Check sheet for the drawn part. Datum: minimum x, y, z corner. Units: mm. A direction names the side the tool comes from. Coordinates: 2 decimals unless noted, no trailing zeros. Write each loop counter-clockwise with the first axis right and the second up, starting at its lowest first coordinate (ties: lowest second). Pieces come first, ordered by that corner, then holes. Notation, with made-up numbers: (81.5, -30) -> (137.5, -30) arc R15 cw to (137.5, -22) -> close; hole circle Ø2 at (-20, 34). An arc over 180 degrees is marked (long way). Answer in a Markdown table with one row per item.
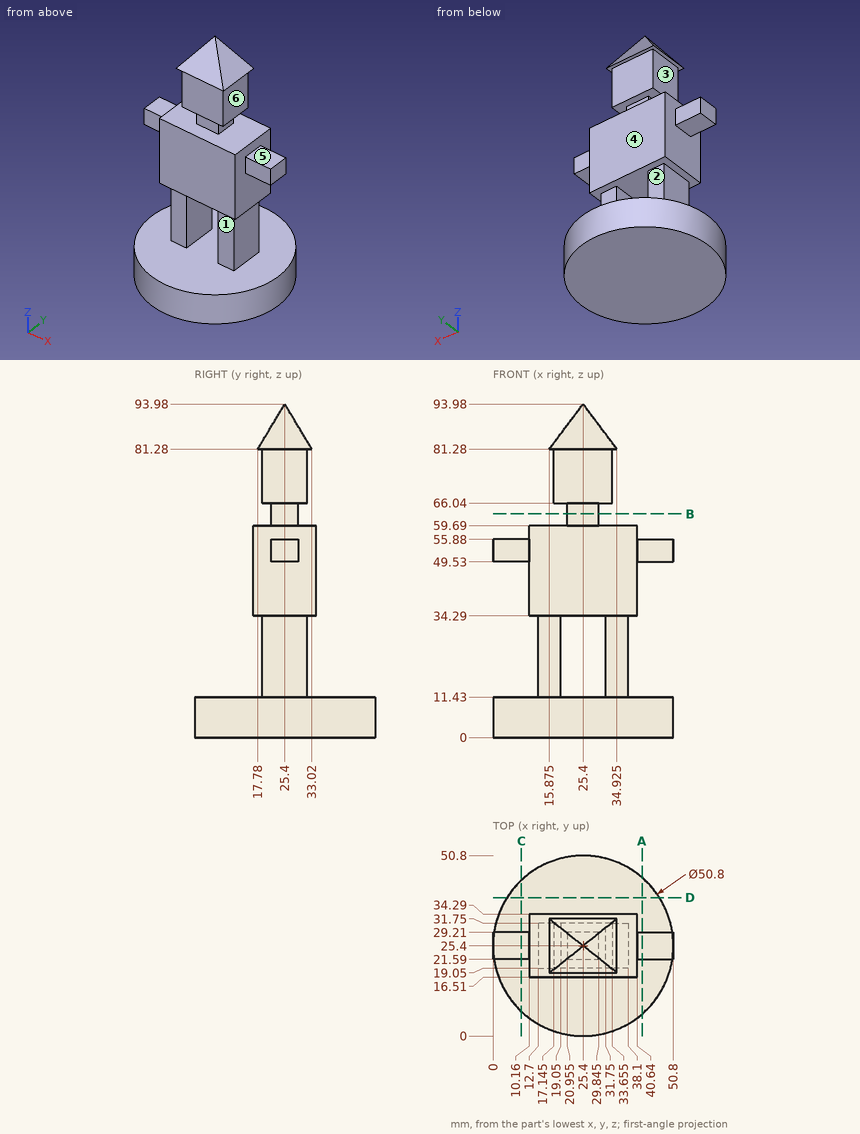
1. Access from +Z, -Z, +X, -X, +Y, -Y to the whole of each face (thin tool, end or side, straight path). Record for the marked faces 1, 2 and 3.
Findings below:
| item | result |
|---|---|
| face 1 | +X, -X, -Y |
| face 2 | +X, -X, +Y |
| face 3 | -X, +Y, -Y |
2. Sectioned sample at C-C, the plane x = 8. Record the cut outline in (y, z).
Findings below:
| item | result |
|---|---|
| outline | (6.9, 0) -> (43.9, 0) -> (43.9, 11.43) -> (6.9, 11.43) -> close; (21.59, 49.53) -> (29.21, 49.53) -> (29.21, 55.88) -> (21.59, 55.88) -> close |
3. Release check for a two-part mould opening along Z. For the marked faces 4, 5 and 6 record: released by +Z, released by -Z, zero draft, split by the parting line, or undercut.
Findings below:
| item | result |
|---|---|
| face 4 | zero draft |
| face 5 | released by +Z |
| face 6 | undercut |
4. Go/stop test with flat-tipped pins: pin 1 (8 mm diameter, centred on x = 34, z = 65, fed in from +Y); pin 2 (7 mm diameter, centred on x = 4, z = 53.5, fed in from +Y); pin 3 (8.5 mm diameter, centred on x = 5, y = 24, fed in from +Z). Record where each tip stops, or that it passes through.
Findings below:
| item | result |
|---|---|
| pin 1 | stops at y = 31.75 |
| pin 2 | stops at y = 29.21 |
| pin 3 | stops at z = 55.88 |
5. Material ranges on probe 1 along X at (y, z) = (23.5, 22.5); probe 2 along Z at (x, y) = (31.5, 27); probe 3 along Y at (x, z) = (25.5, 45.5), recorded low to high. Write a range as from..to.
Findings below:
| item | result |
|---|---|
| probe 1 | x = 12.7..19.05, 31.75..38.1 |
| probe 2 | z = 0..11.43, 34.29..59.69, 66.04..85.85 |
| probe 3 | y = 16.51..34.29 |
6. Sectioned sample at A-A, the plane x = 42. Record the cut outline in (y, z), and give its area (3 significant figures).
Findings below:
| item | result |
|---|---|
| outline | (6.18, 0) -> (44.62, 0) -> (44.62, 11.43) -> (6.18, 11.43) -> close; (21.59, 49.53) -> (29.21, 49.53) -> (29.21, 55.88) -> (21.59, 55.88) -> close |
| area | 488 mm² |
7. Sectioned sample at D-D, the plane y = 39. Record the cut outline in (x, z).
Findings below:
| item | result |
|---|---|
| outline | (3.95, 0) -> (46.85, 0) -> (46.85, 11.43) -> (3.95, 11.43) -> close |
8. Sectioned sample at B-B, the plane z = 63. Record the cut outline in (x, y) (3 decimals), and give its area (3 significant figures).
Findings below:
| item | result |
|---|---|
| outline | (20.955, 21.59) -> (29.845, 21.59) -> (29.845, 29.21) -> (20.955, 29.21) -> close |
| area | 67.7 mm² |
